Geometry check sheet. Reference: the model listing, model coordinates, mm. Face numbers are marked on the shaded views. A direction names the side the tool comes from. Round coordinates to 2 decimals unless told otherwise and drop trailing zeros. Write each loop counter-clockwise with the first axis right and the second up, starting at its lowest first coordinate (ties: lowest second). Pieces come first, ordered by that corner, then holes. Notation, with made-up numbers: (85.25, -37.5) - (134.25, -37.5) arc R13 cw to (134.25, -17.5) - close; hole circle Ø7 at (6.5, 53.25). An arc over 180 degrees is marked (long way). Return JSON: item names as keys, results as strings.
```python
from build123d import *

# Parameters (mm, degrees)
F0_R      = 8
F1_DEPTH  = 20
F2_R      = 4.4
F3_DEPTH  = 20
F4_W      = 34.088476
F4_H      = 19.83197
F4_W_2    = 28.298552
F4_H_2    = 15.987633
F5_DEPTH  = 3
F6_DEPTH  = 3
F7_R      = 8
F8_DEPTH  = 20
F9_R      = 4.4
F10_DEPTH = 20


with BuildPart() as f1:
    # F0 (on Top) → F1 (new body)
    with BuildSketch(Plane.XY):
        Circle(F0_R)
    extrude(amount=F1_DEPTH)

    # F2 (on face) → F3 (cut)
    with BuildSketch(Plane.XY.offset(20)):
        Circle(F2_R)
    extrude(amount=-F3_DEPTH, mode=Mode.SUBTRACT)

    # F4 (on Front) → F5 (join)
    with BuildSketch(Plane.XZ):
        with Locations((-23.512398, 9.915985)):
            Rectangle(F4_W, F4_H)
        with Locations((-23.873756, 9.765204)):
            Rectangle(F4_W_2, F4_H_2, mode=Mode.SUBTRACT)
    extrude(amount=F5_DEPTH)

    # F4 (on Front) → F6 (join)
    with BuildSketch(Plane.XZ):
        with Locations((-23.512398, 9.915985)):
            Rectangle(F4_W, F4_H)
        with Locations((-23.873756, 9.765204)):
            Rectangle(F4_W_2, F4_H_2, mode=Mode.SUBTRACT)
    extrude(amount=-F6_DEPTH)

    # F7 (on face) → F8 (join)
    with BuildSketch(Plane(origin=(0, 0, 0), x_dir=(1, 0, 0), z_dir=(0, 0, -1))):
        with Locations((-47.696788, 0)):
            Circle(F7_R)
    extrude(amount=-F8_DEPTH)

    # F9 (on face) → F10 (cut)
    with BuildSketch(Plane.XY.offset(20)):
        with Locations((-47.696788, 0)):
            Circle(F9_R)
    extrude(amount=-F10_DEPTH, mode=Mode.SUBTRACT)


solid = f1.part
```
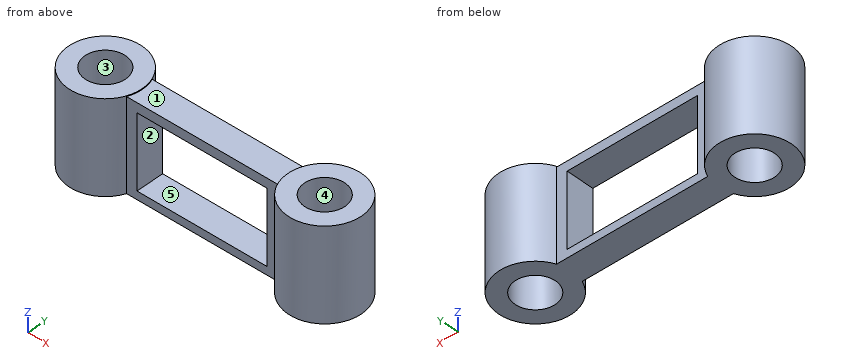
(1) Section check B-B, the plane y = 0. Enter the section's corners in (x, z), plus the area to 3 significant figures.
Response values:
{"outline": "(-55.7, 0) - (-52.1, 0) - (-52.1, 20) - (-55.7, 20) - close; (-43.3, 0) - (-4.4, 0) - (-4.4, 20) - (-8, 20) - (-8, 19.83) - (-39.7, 19.83) - (-39.7, 20) - (-43.3, 20) - close; (4.4, 0) - (8, 0) - (8, 20) - (4.4, 20) - close; hole (-38.02, 1.77) - (-9.72, 1.77) - (-9.72, 17.76) - (-38.02, 17.76) - close", "area": "464 mm^2"}
(2) Section check C-C, the plane x = -24. Enter the section's corners in (y, z), plus the area to 3 significant figures.
Response values:
{"outline": "(-3, 0) - (3, 0) - (3, 1.77) - (-3, 1.77) - close; (-3, 17.76) - (3, 17.76) - (3, 19.83) - (-3, 19.83) - close", "area": "23.1 mm^2"}
(3) Gauge pin test, flat ends, axial feed: pin 1 (4 mm diameter, centred on x = -40, z = 13, fed in from +Y); pin 2 (6 mm diameter, centred on x = -34, z = 12.5, fed in from +Y); pin 3 (8 mm diameter, centred on x = -32, z = 17.5, fed in from +Y); pin 4 (3 mm diameter, centred on x = -40.5, z = 17, fed in from -Y). Record the tip position at first contact, or that the pin passes through.
Response values:
{"pin 1": "stops at y = 5.62", "pin 2": "passes through", "pin 3": "stops at y = 3", "pin 4": "stops at y = -5.62"}
(4) Material ranges on line 1 along X through (y, z) = (1, 7.5); line 2 along X through (y, z) = (2.75, 1.25); line 3 along Y through (x, z) = (0, 12.25), recorded low to high. Write a range as [from, to].
Response values:
{"line 1": "x = [-55.63, -51.98], [-43.41, -38.02], [-9.72, -4.28], [4.28, 7.94]", "line 2": "x = [-55.21, -51.13], [-44.26, -3.43], [3.43, 7.51]", "line 3": "y = [-8, -4.4], [4.4, 8]"}
(5) Release check for a two-part mould opening along Z. For the marked faces 1, 2 and 3 record: pulls with the +Z half, pulls with the -Z half, needs draft (parallel to the pull), parting line crosses it, or undercut.
Response values:
{"face 1": "pulls with the +Z half", "face 2": "undercut", "face 3": "needs draft"}
(6) Section check A-A, the plane z = 8. Enter the section's corners in (x, y), plus the area to 3 significant figures.
Response values:
{"outline": "(-40.28, -3) - (-38.02, -3) - (-38.02, 3) - (-40.28, 3) arc R8 ccw (long way) to start; (-9.72, -3) - (-7.42, -3) arc R8 ccw (long way) to (-7.42, 3) - (-9.72, 3) - close; hole circle Ø8.8 at (-47.7, 0); hole circle Ø8.8 at (0, 0)", "area": "303 mm^2"}
(7) Access from +Z, -Z, +X, -X, +Y, -Y to the whole of each face (thin tool, end or side, straight path). Record for the marked faces 4 and 5.
Response values:
{"face 4": "+Z, -Z", "face 5": "+Y, -Y"}
(8) Section check D-D, the plane y = -3.75. Enter the section's corners in (x, z), plus the area to 3 significant figures.
Response values:
{"outline": "(-54.76, 0) - (-50, 0) - (-50, 20) - (-54.76, 20) - close; (-45.4, 0) - (-40.63, 0) - (-40.63, 20) - (-45.4, 20) - close; (-7.07, 0) - (-2.3, 0) - (-2.3, 20) - (-7.07, 20) - close; (2.3, 0) - (7.07, 0) - (7.07, 20) - (2.3, 20) - close", "area": "381 mm^2"}
